Geometry: final body of the model. Coordinates: model frame, mm. A direction names the side the tool comes from. Give positions to 0.01 mm unless a question says otherwise; leave off trailing zeros. Order: outer loops, then holes, each group sorted by start corner. A loop starts at its lowest first (then second) coordinate and runs counter-clockwise, first axis right, second up. Notation, with made-up numbers: M 31,11 L 54,11 A23 cw 54,33 Z; hole C -4.5,47 d3. An arc over 180 degrees is marked long. Use CSV: the item, a comma, the result in double quotes.
```python
from build123d import *

# Parameters (mm, degrees)
SKETCH2_R                = 5
BOSS_EXTRUDE1_DEPTH      = 20
BOSS_EXTRUDE1_DEPTH_BACK = 20
SKETCH3_R                = 31.686663215
SKETCH4_R                = 8.078892956
SKETCH4_R_2              = 4
CUT_EXTRUDE1_DEPTH       = 8
CHAMFER1_SIZE            = 2


with BuildPart() as part:
    # Sweep1: sweep along a path in Sketch1
    with BuildLine(Plane.XY) as sweep1_path:
        Line((0, 0), (50, 0))
        Line((50, 0), (145.05509307, 31.056871726))
    # Sketch2 → Sweep1 (sweep)
    with BuildSketch(Plane(origin=(0, 0, 0), x_dir=(0, 0, -1), z_dir=(1, 0, 0))):
        Circle(SKETCH2_R)
    sweep(path=sweep1_path.line, transition=Transition.RIGHT)

    # Sketch3 → Boss-Extrude1 (add, two sides: drawn at the far end of the back side and taken through both)
    with BuildSketch(Plane.XY.offset(-BOSS_EXTRUDE1_DEPTH_BACK)):
        with Locations((157.656014811, 51.574343957)):
            Circle(SKETCH3_R)
    extrude(amount=BOSS_EXTRUDE1_DEPTH + BOSS_EXTRUDE1_DEPTH_BACK)

    # Sketch4 → Cut-Extrude1 (cut)
    with BuildSketch(Plane.ZY):
        Circle(SKETCH4_R)
        Circle(SKETCH4_R_2, mode=Mode.SUBTRACT)
    extrude(amount=-CUT_EXTRUDE1_DEPTH, mode=Mode.SUBTRACT)

    # Chamfer1
    chamfer1_edges = [part.edges().sort_by_distance(p)[0] for p in [
        (125.969351596, 51.574343957, -20),
        (125.969351596, 51.574343957, 20),
    ]]
    chamfer(chamfer1_edges, length=CHAMFER1_SIZE)


solid = part.part
```
1. Pin query (flat end, axial travel): pin 1 Ø3 at (x, z) = (149, 4) entering from -Y; pin 2 Ø10 at (x, z) = (25.5, 6.5) entering from +Y. Return the tip coordinate at first contact, or that it passes through.
Answer:
pin 1,"y = 20.71"
pin 2,"y = 4.77"
2. Section A-A, the plane z = 0. Return the cut outline in (x, y), plus the area to 3 significant figures.
Answer:
outline,"M 0,-4 L 8,-4 L 8,-5 L 50.8,-5 L 141.16,24.52 A31.69 ccw long 132.56,32.23 L 49.2,5 L 8,5 L 8,4 L 0,4 Z"
area,"4,550 mm2"
3. Section B-B, the plane z = 9. Return the cut outline in (x, y), plus the area to 3 significant figures.
Answer:
outline,"C 157.66,51.57 d63.37"
area,"3,150 mm2"
4. Reachability of faces 1 (the face through (0, 0, 0)), 2 (the face through (3.944, -3.905, -0.867)) from +Z, -Z, +X, -X, +Y, -Y: full face, straight path, thin tool, end or side. Return the list, or none.
Answer:
face 1,"+Z, -Z, -X, +Y, -Y"
face 2,"-X"
5. Line query: line 1 (X direction, y = 55, z = -10.5); line 2 (Z direction, x = 56, y = 5); line 3 (X direction, y = 77, z = -5). Output: solid intervals per line, ascending.
Answer:
line 1,"126.16 to 189.16"
line 2,"-4.08 to 4.08"
line 3,"138.75 to 176.57"
